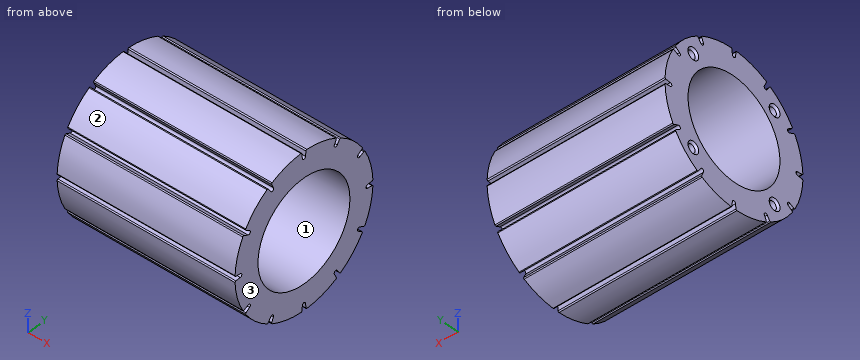
from build123d import *

# Parameters (mm, degrees)
SKETCH008_R           = 30
SKETCH008_R_2         = 20
PAD002_DEPTH          = 70
POCKET_DEPTH          = 70
POLARPATTERN_COUNT    = 12
SKETCH019_R           = 1.6
POCKET001_DEPTH       = 25
POLARPATTERN002_COUNT = 4
CHAMFER_SIZE          = 0.75


with BuildPart() as part:
    # Sketch008 → Pad002 (new body)
    with BuildSketch(Plane.YZ):
        Circle(SKETCH008_R)
        Circle(SKETCH008_R_2, mode=Mode.SUBTRACT)
    extrude(amount=-PAD002_DEPTH)

    # Sketch009 (on Face3 of Pad002) → Pocket (cut)
    with BuildSketch(Plane.YZ):
        with BuildLine():
            ThreePointArc((29.6078316758, 0.8662284607), (29.8735874261, 1.0008336631), (29.9726041, 1.2817969662))
            ThreePointArc((29.9726041, -1.2817969662), (30, 0), (29.9726041, 1.2817969662))
            ThreePointArc((29.9726041, -1.2817969662), (29.8735874261, -1.0008336631), (29.6078316758, -0.8662284607))
            Line((29.6078316758, -0.8662284607), (27.7078316758, -0.7))
            ThreePointArc((27.7078316758, 0.7), (27.0078316758, 0), (27.7078316758, -0.7))
            Line((27.7078316758, 0.7), (29.6078316758, 0.8662284607))
        make_face()
    pocket = extrude(amount=-POCKET_DEPTH, mode=Mode.SUBTRACT)

    # PolarPattern: Pocket ×12 about axis
    polarpattern_axis = Axis((0, 0, 0), (1, 0, 0))
    for i in range(1, POLARPATTERN_COUNT):
        add(pocket.rotate(polarpattern_axis, i * 360 / POLARPATTERN_COUNT), mode=Mode.SUBTRACT)

    # Sketch019 (on Face4 of PolarPattern) → Pocket001 (cut)
    with BuildSketch(Plane(origin=(-70, 0, 0), x_dir=(0, 1, 0), z_dir=(-1, 0, 0))):
        with Locations((17.6776695297, -17.6776695297)):
            Circle(SKETCH019_R)
    pocket001 = extrude(amount=-POCKET001_DEPTH, mode=Mode.SUBTRACT)

    # PolarPattern002: Pocket001 ×4 about axis
    polarpattern002_axis = Axis((-70, 0, 0), (-1, 0, 0))
    for i in range(1, POLARPATTERN002_COUNT):
        add(pocket001.rotate(polarpattern002_axis, i * 360 / POLARPATTERN002_COUNT), mode=Mode.SUBTRACT)

    # Chamfer
    chamfer_edges = [part.edges().sort_by_distance(p)[0] for p in [
        (-70, 17.67767, -16.07767),
        (-70, -16.07767, -17.67767),
        (-70, -17.67767, 16.07767),
        (-70, 16.07767, 17.67767),
    ]]
    chamfer(chamfer_edges, length=CHAMFER_SIZE)


solid = part.part
Can you work these out from the model? Positions are in its coordinate system, mm. Face numbers are marked on the shaded views. Coordinates: 2 decimals unless noted, no trailing zeros. Loops run counter-clockwise (first coordinate to the right, second up) from the corner with the lowest first, then second, coordinate; pieces in that order, holes last. Notation, with made-up numbers: (57.5, 39) - (65.5, 39) arc R18 cw to (65.5, 60) - close; hole circle Ø3 at (54.25, 12.25). An arc over 180 degrees is marked (long way). Put each result on its own line as item: value. Start each with the question number.
Item 1: If I drill on line 1 along Z through (x, y) = (-12.5, -25); line 2 along Z through (x, y) = (-20, 0); line 3 along Z through (x, y) = (-50, -16.5), over which ranges is the centre line in solid material (lowest first)?
Item 2: Suppose I cut it at D-D (y = -21). Please give me the cut outline in (x, z).
Item 3: Suppose I cut it at A-A (y = 6). Please give me the cut outline in (x, z).
Item 4: For pin 1 (2 mm diameter, centred on x = -33.5, y = -5.5, fed in from +Z); pin 2 (2.5 mm diameter, centred on y = 18, z = 18, fed in from -X); pin 3 (1 mm diameter, centred on x = -59, y = -18.5, fed in from +Z), each with a flat end and sliding along its axis, tell me the tip position at first contact or that it passes through.
Item 5: Suppose I cut it at C-C (x = -51.5). State how many separate pieces and enclosed holes the cut face has, and give its area (3 significant figures).
Item 6: If we mould it in two halves opening along Z, with no side actions, what happens to the marked faces 1, 2 and 3? For each: +Z half, -Z half, draft (parallel to the pull), parting line (faces both ways), or undercut.
Item 7: Suppose I cut it at B-B (z = 10.5). Please give me the cut outline in (x, y).
Here are the results:
1. line 1: -16.58 to -15.41, -13.55 to 13.55, 15.41 to 16.58
1. line 2: -27.01 to -20, 20 to 27.01
1. line 3: -25.05 to -18.76, -16.59 to -11.3, 11.3 to 16.59, 18.76 to 25.05
2. outline: (-70, -21.42) - (0, -21.42) - (0, 21.42) - (-70, 21.42) - close
3. outline: (-70, -29.39) - (0, -29.39) - (0, -19.08) - (-70, -19.08) - close; (-70, 19.08) - (0, 19.08) - (0, 29.39) - (-70, 29.39) - close
4. pin 1: z = 29.66
4. pin 2: x = -69.36
4. pin 3: z = 24
5. separate pieces: 1
5. enclosed holes: 5
5. area: 1,480 mm²
6. face 1: undercut
6. face 2: +Z half
6. face 3: draft
7. outline: (-70, -28.1) - (0, -28.1) - (0, -17.02) - (-70, -17.02) - close; (-70, 17.02) - (0, 17.02) - (0, 28.1) - (-70, 28.1) - close
